Input: part model. Units: mm. Frame: model coordinates. Face numbers are marked on the shaded views. A direction names the side the tool comes from. Coordinates: 2 decimals unless noted, no trailing zeros. Loops run counter-clockwise (first coordinate to the right, second up) from the corner with the lowest first, then second, coordinate; pieces in that order, holes last. Notation, with made-up numbers: (60, -33) -> (79, -33) arc R33 ccw to (79, -2) -> close; hole circle Ø8 at (19.25, -39.75). An arc over 180 degrees is marked (long way). Answer as a JSON object with one key per item and string values.
from build123d import *

# Parameters (mm, degrees)
F0_W     = 76.2
F0_H     = 101.6
F1_DEPTH = 76.2
F2_R     = 25.777138
F3_DEPTH = 25.4


with BuildPart() as f1:
    # F0 (on Front) → F1 (new body)
    with BuildSketch(Plane.XZ):
        with Locations((38.1, 50.8)):
            Rectangle(F0_W, F0_H)
    extrude(amount=-F1_DEPTH)

    # F2 (on face) → F3 (cut)
    with BuildSketch(Plane(origin=(0, 76.2, 0), x_dir=(-1, 0, 0), z_dir=(0, 1, 0))):
        with Locations((-35.715438, 61.196949)):
            Circle(F2_R)
    extrude(amount=-F3_DEPTH, mode=Mode.SUBTRACT)


solid = f1.part
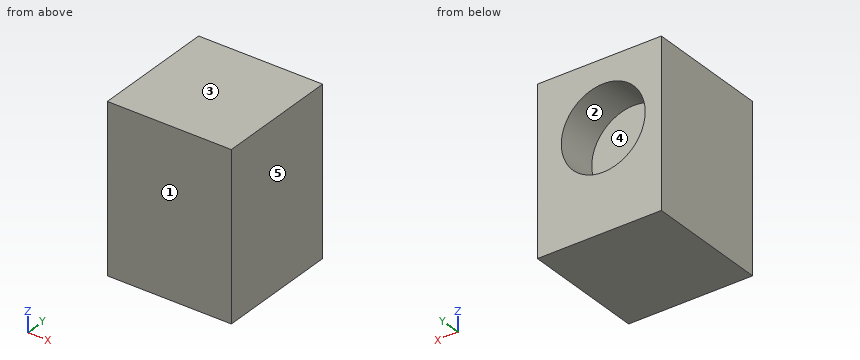
1. Line query: line 1 along Y through (x, z) = (49, 62); line 2 along X through (y, z) = (59.5, 76); line 3 along X through (y, z) = (68.5, 83.5). Output: solid intervals per line, ascending.
Reply:
{"line 1": "y = 0 to 50.8", "line 2": "x = 0 to 14.61, 56.82 to 76.2", "line 3": "x = 0 to 22.79, 48.64 to 76.2"}
2. Mould query, pull axis Z, two halves, no side actions, for the marked faces 3, 4 and 5. Classes: pulls with the +Z half, pulls with the -Z half, needs draft (parallel to the pull), parting line crosses it, or undercut.
Reply:
{"face 3": "pulls with the +Z half", "face 4": "undercut", "face 5": "needs draft"}
3. Section query B-B (x = 51). Return loops of the section in (y, z).
Reply:
{"outline": "(0, 0) -> (76.2, 0) -> (76.2, 40.44) -> (50.8, 40.44) -> (50.8, 81.95) -> (76.2, 81.95) -> (76.2, 101.6) -> (0, 101.6) -> close"}
4. Access query for the marked faces 1 and 2. Directions: +Z, -Z, +X, -X, +Y, -Y. A direction counts if a zero-diameter tool reaches every point of the face in a straight line with its end or side. Return the directions, or none.
Reply:
{"face 1": "+Z, -Z, +X, -X, -Y", "face 2": "+Y"}
5. Section query C-C (z = 59.5). Return loops of the section in (x, y), plus the area to 3 significant figures.
Reply:
{"outline": "(0, 0) -> (76.2, 0) -> (76.2, 76.2) -> (61.44, 76.2) -> (61.44, 50.8) -> (9.99, 50.8) -> (9.99, 76.2) -> (0, 76.2) -> close", "area": "4,500 mm2"}
6. Section query A-A (y = 61). Return loops of the section in (x, z), plus the area to 3 significant figures.
Reply:
{"outline": "(0, 0) -> (76.2, 0) -> (76.2, 101.6) -> (0, 101.6) -> close; hole circle Ø51.55 at (35.72, 61.2)", "area": "5,650 mm2"}
